```python
from build123d import *

# Parameters (mm, degrees)
SKETCH1_R                 = 2.2
BOSS_EXTRUDE1_DEPTH       = 6
SKETCH4_W                 = 30
SKETCH4_H                 = 6
BOSS_EXTRUDE3_DEPTH       = 20
SKETCH5_R                 = 10
SKETCH5_R_2               = 4.25
BOSS_EXTRUDE4_DEPTH       = 20
CUT_EXTRUDE1_START        = -20
SKETCH7_R                 = 4.25
CUT_EXTRUDE1_DEPTH        = 20
RIB1_REACH                = 118.934
SKETCH8_WALL_W            = 247.402128672
SKETCH8_WALL_H            = 5
CIRPATTERN2_COUNT         = 2
CIRPATTERN2_ANGLE         = 180
LPATTERN3_COUNT           = 2
LPATTERN3_PITCH           = 68.3
LPATTERN3_COPY_1_REACH    = 118.934
LPATTERN3_COPY_1_SKETCH_W = 247.402128672
LPATTERN3_COPY_1_SKETCH_H = 5
FILLET4_R                 = 1
CUT_EXTRUDE2_START        = -20
SKETCH9_R                 = 4.25
CUT_EXTRUDE2_DEPTH        = 20


with BuildPart() as part:
    # Sketch1 → Boss-Extrude1 (new body)
    with BuildSketch(Plane.XY):
        Polygon((-15, 51.15), (15, 51.15), (15, -17.15), (30, -17.15), (30, -51.15), (15, -51.15), (-15, -51.15), (-30, -51.15), (-30, -17.15), (-15, -17.15), align=None)
        with Locations((9, 46.15)):
            Circle(SKETCH1_R, mode=Mode.SUBTRACT)
        with Locations((-9, 46.15)):
            Circle(SKETCH1_R, mode=Mode.SUBTRACT)
        with Locations((-9, 22.15)):
            Circle(SKETCH1_R, mode=Mode.SUBTRACT)
        with Locations((9, 22.15)):
            Circle(SKETCH1_R, mode=Mode.SUBTRACT)
        with Locations((-6, -22.15)):
            Circle(SKETCH1_R, mode=Mode.SUBTRACT)
        with Locations((-24, -22.15)):
            Circle(SKETCH1_R, mode=Mode.SUBTRACT)
        with Locations((-24, -46.15)):
            Circle(SKETCH1_R, mode=Mode.SUBTRACT)
        with Locations((-6, -46.15)):
            Circle(SKETCH1_R, mode=Mode.SUBTRACT)
        with Locations((6, -22.15)):
            Circle(SKETCH1_R, mode=Mode.SUBTRACT)
        with Locations((24, -22.15)):
            Circle(SKETCH1_R, mode=Mode.SUBTRACT)
        with Locations((6, -46.15)):
            Circle(SKETCH1_R, mode=Mode.SUBTRACT)
        with Locations((24, -46.15)):
            Circle(SKETCH1_R, mode=Mode.SUBTRACT)
    extrude(amount=BOSS_EXTRUDE1_DEPTH)

    # Sketch4 → Boss-Extrude3 (add)
    with BuildSketch(Plane(origin=(0, 51.15, 0), x_dir=(1, 0, 0), z_dir=(0, 1, 0))):
        with Locations((0, -3)):
            Rectangle(SKETCH4_W, SKETCH4_H)
    extrude(amount=BOSS_EXTRUDE3_DEPTH)

    # Sketch5 → Boss-Extrude4 (add)
    with BuildSketch(Plane.XY.offset(6)):
        with Locations((0, 61.15)):
            Circle(SKETCH5_R)
        with Locations((0, 61.15)):
            Circle(SKETCH5_R_2, mode=Mode.SUBTRACT)
    boss_extrude4 = extrude(amount=-BOSS_EXTRUDE4_DEPTH)

    # Sketch7 → Cut-Extrude1 (cut)
    with BuildSketch(Plane(origin=(0, 0, 0), x_dir=(-1, 0, 0), z_dir=(0, 0, -1)).offset(CUT_EXTRUDE1_START)):
        with Locations(Location((0, 61.15, 0), (0, 0, 180))):
            Circle(SKETCH7_R)
    extrude(amount=CUT_EXTRUDE1_DEPTH, mode=Mode.SUBTRACT)

    # Sketch8 wall → Rib1 (add, up to next)
    with BuildSketch(Plane(origin=(12.5, 61, -5.196726493), x_dir=(-0.433516092302, 0, -0.901145824889), z_dir=(-0.901145824889, 0, 0.433516092302)), mode=Mode.PRIVATE) as rib1_sk1:
        Rectangle(SKETCH8_WALL_W, SKETCH8_WALL_H)
    rib1_tool1 = extrude(rib1_sk1.sketch, amount=RIB1_REACH, mode=Mode.PRIVATE) - part.part
    rib1 = rib1_tool1.solids().sort_by_distance((12.5, 61, -5.196726493))[0]
    add(rib1)

    # CirPattern2: Rib1 ×2 about axis
    cirpattern2_axis = Axis((0, 61.15, -14), (0, 0, 1))
    for i in range(1, CIRPATTERN2_COUNT):
        add(rib1.rotate(cirpattern2_axis, i * CIRPATTERN2_ANGLE / (CIRPATTERN2_COUNT - 1)))

    # LPattern3: Boss-Extrude4, Rib1 ×2
    with Locations(*[(0, -i * LPATTERN3_PITCH, 0) for i in range(1, LPATTERN3_COUNT)]):
        add(boss_extrude4)
        add(rib1)

    # LPattern3 copy 1 sketch → LPattern3 copy 1 (add, up to next)
    with BuildSketch(Plane(origin=(-12.5, -7, -5.196726493), x_dir=(0.433516092302, 3.0272266927212608e-15, -0.901145824889), z_dir=(0.901145824889, 6.292667662352691e-15, 0.433516092302)), mode=Mode.PRIVATE) as lpattern3_copy_1_sk1:
        Rectangle(LPATTERN3_COPY_1_SKETCH_W, LPATTERN3_COPY_1_SKETCH_H)
    lpattern3_copy_1_tool1 = extrude(lpattern3_copy_1_sk1.sketch, amount=LPATTERN3_COPY_1_REACH, mode=Mode.PRIVATE) - part.part
    add(lpattern3_copy_1_tool1.solids().sort_by_distance((-12.5, -7, -5.196726493))[0])

    # Fillet4
    fillet4_edges = [part.edges().sort_by_distance(p)[0] for p in [
        (12.359976852, 63.5, 0),
        (9.719953704, 63.5, -5.487791295),
        (9.64248412, 58.5, -5.568308943),
        (12.32124206, 58.5, 0),
        (-9.64248412, 63.8, -5.568308943),
        (-12.32124206, 63.8, 0),
        (-12.359976852, 58.8, 0),
        (-9.719953704, 58.8, -5.487791295),
        (12.359976852, -4.8, 0),
        (9.64248412, -9.8, -5.568308943),
        (9.719953704, -4.8, -5.487791295),
        (12.32124206, -9.8, 0),
        (-9.64248412, -4.5, -5.568308943),
        (-12.359976852, -9.5, 0),
        (-9.719953704, -9.5, -5.487791295),
        (-12.32124206, -4.5, 0),
    ]]
    fillet(fillet4_edges, radius=FILLET4_R)

    # Sketch9 → Cut-Extrude2 (cut)
    with BuildSketch(Plane(origin=(0, 0, 0), x_dir=(-1, 0, 0), z_dir=(0, 0, -1)).offset(CUT_EXTRUDE2_START)):
        with Locations(Location((0, -7.15, 0), (0, 0, 180))):
            Circle(SKETCH9_R)
    extrude(amount=CUT_EXTRUDE2_DEPTH, mode=Mode.SUBTRACT)


solid = part.part
```
Verification items for the finished model (mm, model axes). A direction names the side the tool comes from. Round coordinates to 2 decimals unless told otherwise and drop trailing zeros. Write each loop counter-clockwise with the first axis right and the second up, starting at its lowest first coordinate (ties: lowest second). Pieces come first, ordered by that corner, then holes. Notation, with made-up numbers: (72.25, -34) - (105.25, -34) arc R37 ccw to (105.25, 4) - close; hole circle Ø6 at (73.25, 47.25). An arc over 180 degrees is marked (long way). Answer as a JSON object with one key per item and string values. Group by question number.
Q1. Section check D-D, the plane x = 24. Enter the section's corners in (y, z).
Q2. Thickness scan on line 1 (Y direction, x = -9, z = 2.15); line 2 (Y direction, x = 0, z = 1.45); line 3 (Y direction, x = 2, z = -4.75). Record the ranges inside material, lowest first.
Q3. Section check C-C, the plane y = -46.15. Enter the section's corners in (x, z).
Q4. Go/stop test with flat-tipped pins: pin 1 Ø6 at (y, z) = (-18.5, -7.5) entering from -X; pin 2 Ø10 at (x, y) = (1, 27) entering from -Z; pin 3 Ø2 at (x, z) = (-12, -6) entering from +Y; pin 4 Ø8 at (x, y) = (-5, -19.5) entering from -Z. Record where each tip stops, or that it passes through.
Q5. Mould release check, pull along Y, two halves, no side actions. Record for faces 4 (the flat face through (4, -9, -14)), 5 (the cylindrical face through (-6.477, -48.298, 2.958)), 6 (the flat face through (22, -17.15, 3)): released by +Y, released by -Y, zero draft, split by the parting line, or undercut.
Q6. Section check B-B, the plane z = -4.5. Enter the section's corners in (x, y).
Q7. Section check A-A, the plane y = 46.15. Enter the section's corners in (x, z).
Q8. Tool access check on faces 1 (the flat face through (-12, -9.5, -4)), 2 (the cylindrical face through (4.614, 52.278, -6.902)), 3 (the flat face through (15, 26, 3)). Record the directions out of +Z, -Z, +X, -X, +Y, -Y that give a thin tool (end or side, any length) a straight path to the whole face; none if there is none.
Found:
{
 "1": {"outline": "(-51.15, 0) - (-48.35, 0) - (-48.35, 6) - (-51.15, 6) - close; (-43.95, 0) - (-24.35, 0) - (-24.35, 6) - (-43.95, 6) - close; (-19.95, 0) - (-17.15, 0) - (-17.15, 6) - (-19.95, 6) - close"},
 "2": {"line 1": "y = -51.15 to 19.95, 24.35 to 43.95, 48.35 to 71.15", "line 2": "y = -51.15 to -11.4, -2.9 to 56.9, 65.4 to 71.15", "line 3": "y = -16.95 to -10.9, -3.4 to 2.65, 51.35 to 57.4, 64.9 to 70.95"},
 "3": {"outline": "(-30, 0) - (-26.2, 0) - (-26.2, 6) - (-30, 6) - close; (-21.8, 0) - (-8.2, 0) - (-8.2, 6) - (-21.8, 6) - close; (-3.8, 0) - (3.8, 0) - (3.8, 6) - (-3.8, 6) - close; (8.2, 0) - (21.8, 0) - (21.8, 6) - (8.2, 6) - close; (26.2, 0) - (30, 0) - (30, 6) - (26.2, 6) - close"},
 "4": {"pin 1": "stops at x = -5.5", "pin 2": "stops at z = 0", "pin 3": "stops at y = 63.8", "pin 4": "stops at z = -14"},
 "5": {"face 4": "zero draft", "face 5": "undercut", "face 6": "released by +Y"},
 "6": {"outline": "(-12.84, -9.5) - (-10.48, -9.5) arc R1 cw to (-9.52, -10.2) arc R10 ccw to (9.43, -10.47) arc R1 cw to (10.38, -9.8) - (12.84, -9.8) - (12.84, -4.8) - (10.48, -4.8) arc R1 cw to (9.52, -4.1) arc R10 ccw to (-9.43, -3.83) arc R1 cw to (-10.38, -4.5) - (-12.84, -4.5) - close; (-12.84, 58.8) - (-10.48, 58.8) arc R1 cw to (-9.52, 58.1) arc R10 ccw to (9.43, 57.83) arc R1 cw to (10.38, 58.5) - (12.84, 58.5) - (12.84, 63.5) - (10.48, 63.5) arc R1 cw to (9.52, 64.2) arc R10 ccw to (-9.43, 64.47) arc R1 cw to (-10.38, 63.8) - (-12.84, 63.8) - close; hole circle Ø8.5 at (0, -7.15); hole circle Ø8.5 at (0, 61.15)"},
 "7": {"outline": "(-15, 0) - (-11.2, 0) - (-11.2, 6) - (-15, 6) - close; (-6.8, 0) - (6.8, 0) - (6.8, 6) - (-6.8, 6) - close; (11.2, 0) - (15, 0) - (15, 6) - (11.2, 6) - close"},
 "8": {"face 1": "-Z, -X, -Y", "face 2": "-Z", "face 3": "+Z, -Z, +X, +Y"}
}
